Build history of the part. All positions in model axes, mm. Coordinates: 2 decimals unless noted, no trailing zeros. Loops run counter-clockwise (first coordinate to the right, second up) from the corner with the lowest first, then second, coordinate; pieces in that order, holes last.
Item 1: Cut at A-A (z = 144). List the corners of the cut face in (x, y), and give its area (3 significant figures).
Item 2: Cut at B-B (y = 3.5). List the corners of the cut face in (x, z), and give its area (3 significant figures).
Item 3: Drill centre lines: line 1 along Z through (x, y) = (7.5, 8.7); line 2 along X through (y, z) = (1.4, 45); line 3 along Y through (x, z) = (3.5, 46). Where is each one in solid material? Low to high.
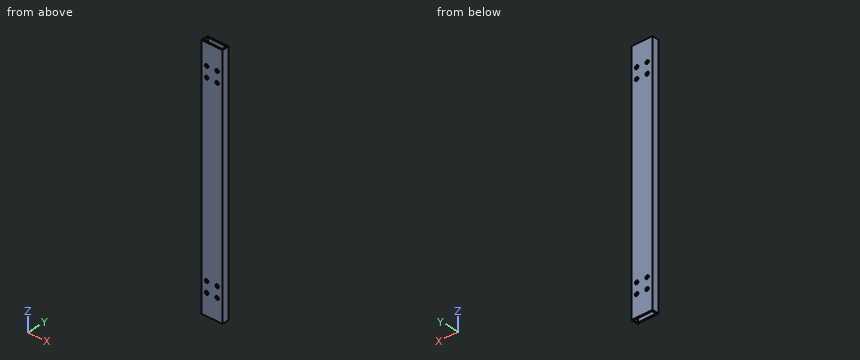
Autodesk Inventor part; units mm, degrees
ref_plane "YZ Plane" through (0, 0, 0) normal (1, 0, 0) x (0, 1, 0)
ref_plane "XZ Plane" through (0, 0, 0) normal (0, 1, 0) x (-1, 0, 0)
ref_plane "XY Plane" through (0, 0, 0) normal (0, 0, 1) x (1, 0, 0)
sketch "Sketch2" plane through (0, 0, 0) normal (0, 0, 1) x (1, 0, 0)
  line L0 (0, 0) -> (30, 0)
  line L1 (30, 0) -> (30, 10)
  line L2 (30, 10) -> (0, 10)
  line L3 (0, 10) -> (0, 0)
  line L4 (2.0014, 2) -> (28.0014, 2)
  line L5 (28.0014, 2) -> (28.0014, 8)
  line L6 (28.0014, 8) -> (2.0014, 8)
  line L7 (2.0014, 8) -> (2.0014, 2)
  dimension "d0" = 30
  dimension "d1" = 10
  dimension "d2" = 26
  dimension "d3" = 6
extrude "Extrusion1" add sketch "Sketch2" along normal blind 350
sketch "Sketch3" plane through (0, 10, 0) normal (0, 1, 0) x (1, 0, 0)
  circle A0 centre (7.5, -30) radius 2.5
  circle A1 centre (22.5, -30) radius 2.5
  circle A2 centre (7.5, -45) radius 2.5
  circle A3 centre (22.5, -45) radius 2.5
  circle A4 centre (7.5, -320) radius 2.5
  circle A5 centre (22.5, -320) radius 2.5
  circle A6 centre (7.5, -305) radius 2.5
  circle A7 centre (22.5, -305) radius 2.5
  point P0 (0, 0)
  dimension "d6" = 5
  dimension "d7" = 5
  dimension "d8" = 5
  dimension "d9" = 5
  dimension "d10" = 5
  dimension "d11" = 5
  dimension "d12" = 5
  dimension "d13" = 5
extrude "Extrusion2" cut sketch "Sketch3" against normal blind 169.1125
properties part number "long_frame" material "Aluminum 6061"
Filled sheet:
1. outline: (0, 0) - (30, 0) - (30, 10) - (0, 10) - close; hole (2, 2) - (28, 2) - (28, 8) - (2, 8) - close
1. area: 144 mm2
2. outline: (0, 0) - (2, 0) - (2, 350) - (0, 350) - close; (28, 0) - (30, 0) - (30, 350) - (28, 350) - close
2. area: 1,400 mm2
3. line 1: z = 0 to 27.5, 32.5 to 42.5, 47.5 to 302.5, 307.5 to 317.5, 322.5 to 350
3. line 2: x = 0 to 5, 10 to 20, 25 to 30
3. line 3: y = 0 to 2, 8 to 10
